from build123d import *

# Parameters (mm, degrees)
F0_W      = 29.3072769418
F0_H      = 51.8513377756
F1_DEPTH  = 25.4
F2_R      = 6.2145404026
F2_R_2    = 6.5329388007
F3_DEPTH  = 73.914
F4_W      = 13.2390642539
F4_H      = 29.6439919621
F5_DEPTH  = 36.322
F6_R      = 6.9321854406
F7_DEPTH  = 18.034
F9_DEPTH  = 24.892
F10_R     = 3.6433318827
F11_DEPTH = 55.88


with BuildPart() as f1:
    # F0 (on Top) → F1 (new body)
    with BuildSketch(Plane.XY):
        with Locations((0.6441161968, -0.3612739965)):
            Rectangle(F0_W, F0_H)
        with BuildLine():
            Line((15.2977546677, -26.2869428843), (-14.0095222741, -26.2869428843))
            ThreePointArc((-14.0095222741, -26.2869428843), (0.6441161968, -40.9405813552), (15.2977546677, -26.2869428843))
        make_face()
        with BuildLine():
            ThreePointArc((15.2977546677, 25.5643948913), (0.6441161968, 40.2180333622), (-14.0095222741, 25.5643948913))
            Line((-14.0095222741, 25.5643948913), (15.2977546677, 25.5643948913))
        make_face()
    extrude(amount=F1_DEPTH)

    # F2 (on Top) → F3 (cut)
    with BuildSketch(Plane.XY):
        with Locations((0, -29.2122848332)):
            Circle(F2_R)
        with Locations((0, 29.2122848332)):
            Circle(F2_R_2)
    extrude(amount=F3_DEPTH, mode=Mode.SUBTRACT)

    # F4 (on Top) → F5 (join)
    with BuildSketch(Plane.XY):
        with Locations((0.1439033076, 2.0146397874)):
            Rectangle(F4_W, F4_H)
    extrude(amount=F5_DEPTH)

    # F6 (on Front) → F7 (join, symmetric)
    with BuildSketch(Plane.XZ):
        with Locations((0, 35.4015231133)):
            Circle(F6_R)
    extrude(amount=F7_DEPTH, both=True)

    # F8 (on Right) → F9 (cut, symmetric)
    with BuildSketch(Plane.YZ):
        with BuildLine():
            Line((-1.3480700781, 42.4513481557), (-5.6122136302, 42.4513481557))
            Line((-5.6122136302, 42.4513481557), (-5.6122136302, 35.2562069893))
            ThreePointArc((-5.6122136302, 35.2562069893), (-4.4661066114, 39.4381017942), (-1.3480700781, 42.4513481557))
        make_face()
        with BuildLine():
            ThreePointArc((6.5285728542, 42.4513481557), (2.590251388, 43.4586720075), (-1.3480700781, 42.4513481557))
            Line((-1.3480700781, 42.4513481557), (6.5285728542, 42.4513481557))
        make_face()
        with BuildLine():
            Line((6.5285728542, 42.4513481557), (-1.3480700781, 42.4513481557))
            ThreePointArc((-1.3480700781, 42.4513481557), (-4.4661066114, 39.4381017942), (-5.6122136302, 35.2562069893))
            Line((-5.6122136302, 35.2562069893), (10.7927164063, 35.2562069893))
            ThreePointArc((10.7927164063, 35.2562069893), (9.6466093875, 39.4381017942), (6.5285728542, 42.4513481557))
        make_face()
        with BuildLine():
            Line((10.7927164063, 35.2562069893), (-5.6122136302, 35.2562069893))
            ThreePointArc((-5.6122136302, 35.2562069893), (2.590251388, 27.053741971), (10.7927164063, 35.2562069893))
        make_face()
        with BuildLine():
            Line((10.7927164063, 42.4513481557), (6.5285728542, 42.4513481557))
            ThreePointArc((6.5285728542, 42.4513481557), (9.6466093875, 39.4381017942), (10.7927164063, 35.2562069893))
            Line((10.7927164063, 35.2562069893), (10.7927164063, 42.4513481557))
        make_face()
    extrude(amount=F9_DEPTH, both=True, mode=Mode.SUBTRACT)

    # F10 (on Front) → F11 (cut, symmetric)
    with BuildSketch(Plane.XZ):
        with Locations((0, 36.1196212471)):
            Circle(F10_R)
    extrude(amount=F11_DEPTH, both=True, mode=Mode.SUBTRACT)


solid = f1.part
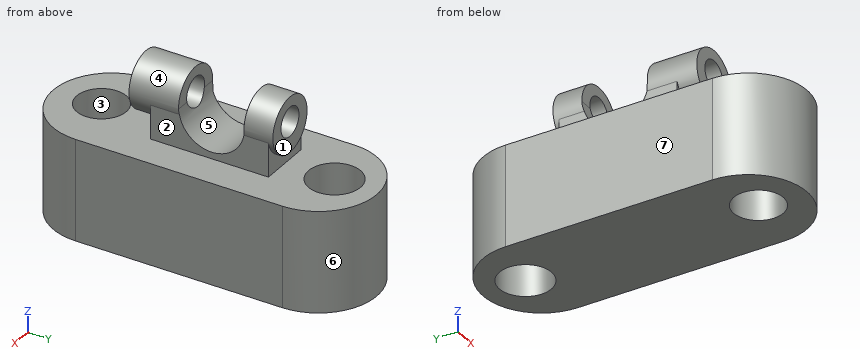
Work out the finished part from the listing and answer in its coordinate system (mm). Face numbers are marked on the shaded views. A direction names the side the tool comes from. Give positions to 0.01 mm unless a question says otherwise; leave off trailing zeros. Order: outer loops, then holes, each group sorted by start corner. A loop starts at its lowest first (then second) coordinate and runs counter-clockwise, first axis right, second up. Notation, with made-up numbers: (64, -21) -> (102, -21) arc R17 ccw to (102, 10) -> close; hole circle Ø2 at (15, -40). An arc over 180 degrees is marked (long way). Answer as a JSON object with one key per item and string values. Group by question number.
1. Section A-A on x = -1.5 is taken. Count the separate pieces of the cut face and the enclosed holes in it, plus the area to 3 significant figures.
2. Section D-D on x = -11 is taken. Determine the outline of the cut face in (y, z).
3. Flat-ended cylindrical pins translate along their axes: pin 1 Ø3.5 at (x, z) = (-1.5, 39) entering from -Y; pin 2 Ø1 at (x, z) = (-1, 17.5) entering from +Y; pin 3 Ø3 at (x, y) = (9.5, 12.5) entering from +Z. Find the tip coordinate at first contact, or state that the pin passes through.
4. The mould has two halves that part along Y. Classify the marked faces 5, 6 and 7: released by +Y, released by -Y, zero draft, split by the parting line, or undercut.
5. Section C-C on z = 4.5 is taken. Determine the outline of the cut face in (x, y), plus the area to 3 significant figures.
6. A tool of negligible diameter and unlimited length cuts with its end or side. For the marked faces 1, 2, 3 and 4, from which of +Z, -Z, +X, -X, +Y, -Y can it reach the whole face along a straight path? Write none if from no direction.
7. Section B-B on y = 27 is taken. Determine the outline of the cut face in (x, z).
8. Consider line 1 along Y through (x, z) = (0, 7.25); line 2 along Z through (x, y) = (0, -14); line 3 along Y through (x, z) = (5, 12.5). Determine where each line is inside the solid, lowest interval first. Write a range as [from, to].
Result sheet:
{
 "1": {"separate pieces": "5", "enclosed holes": "0", "area": "1,660 mm^2"},
 "2": {"outline": "(-35.18, 0) -> (34.46, 0) -> (34.46, 25.4) -> (-35.18, 25.4) -> close"},
 "3": {"pin 1": "stops at y = -18.03", "pin 2": "stops at y = 40.17", "pin 3": "stops at z = 25.4"},
 "4": {"face 5": "undercut", "face 6": "released by +Y", "face 7": "zero draft"},
 "5": {"outline": "(-14.01, -26.29) arc R14.65 ccw to (15.3, -26.29) -> (15.3, 25.56) arc R14.65 ccw to (-14.01, 25.56) -> close; hole circle Ø13.07 at (0, 29.21); hole circle Ø12.43 at (0, -29.21)", "area": "1,940 mm^2"},
 "6": {"face 1": "+Z, +X, -X, +Y", "face 2": "+X, +Y, -Y", "face 3": "+Z, -Z", "face 4": "-Y"},
 "7": {"outline": "(-13.94, 0) -> (-6.15, 0) -> (-6.15, 25.4) -> (-13.94, 25.4) -> close; (6.15, 0) -> (15.23, 0) -> (15.23, 25.4) -> (6.15, 25.4) -> close"},
 "8": {"line 1": "y = [-40.93, -35.43], [-23, 22.68], [35.75, 40.2]", "line 2": "z = [0, 25.4], [28.47, 32.48], [39.76, 42.33]", "line 3": "y = [-40.28, -32.9], [-25.52, 25.01], [33.42, 39.56]"}
}
